Input: part model. Units: mm. Frame: model coordinates. Face numbers are marked on the shaded views. A direction names the side the tool comes from. Coordinates: 2 decimals unless noted, no trailing zeros. Write each loop counter-clockwise with the first axis right and the second up, starting at its lowest first coordinate (ties: lowest second). Pieces come first, ordered by that corner, then holes. Notation, with made-up numbers: (52.5, 79.25) - (63.5, 79.25) arc R14 cw to (63.5, 92.25) - close; hole circle Ø11 at (58.5, -35). An arc over 180 degrees is marked (long way). Put each result on its own line as item: value. Start each with the question number.
1. Pin query (flat end, axial travel): pin 1 (6 mm diameter, centred on x = -10, y = 9.5, fed in from -Z); pin 2 (3 mm diameter, centred on x = 17.5, z = 0, fed in from +Y); pin 3 (5 mm diameter, centred on x = 8, z = -10, fed in from +Y); pin 4 (5 mm diameter, centred on y = 6.5, z = 7.5, fed in from +X). Return the tip coordinate at first contact, or that it passes through.
2. Cut plane B-B, the plane x = -17. Return loops of the section in (y, z).
3. Access query for the marked faces 1 and 2. Directions: +Z, -Z, +X, -X, +Y, -Y. A direction counts if a zero-diameter tool reaches every point of the face in a straight line with its end or side. Return the directions, or none.
4. Cut plane A-A, the plane z = 0. Return loops of the section in (x, y), and give its area (3 significant figures).
5. Cut plane D-D, the plane z = 11.5. Return loops of the section in (x, y).
6. Cut plane C-C, the plane x = -4.5. Return loops of the section in (y, z), and give its area (3 significant figures).
7. Line query: line 1 (Y direction, x = -5, z = -10); line 2 (Z direction, x = 17.5, y = 0.75); line 3 (Y direction, x = 18.5, z = 5). Output: solid intervals per line, ascending.
from build123d import *

# Parameters (mm, degrees)
SKETCH_1_R      = 16.1
EXTRUDE_1_DEPTH = 1
SKETCH_2_R      = 13.5
EXTRUDE_2_DEPTH = 9
HOLE_WIZARD_1_D = 4
FILLET_1_R      = 10


with BuildPart() as part:
    # 草图1 → 凸台-拉伸1 (new body)
    with BuildSketch(Plane(origin=(0, 0, 0), x_dir=(1, 0, 0), z_dir=(0, 1, 0))):
        with BuildLine():
            Line((-23.5, 16.1), (-23.5, -16.1))
            Line((-23.5, -16.1), (0, -16.1))
            ThreePointArc((0, -16.1), (-16.1, 0), (0, 16.1))
            Line((0, 16.1), (-23.5, 16.1))
        make_face()
        Circle(SKETCH_1_R)
        with BuildLine():
            ThreePointArc((16.1, 0), (11.384419177, -11.384419177), (0, -16.1))
            Line((0, -16.1), (23.5, -16.1))
            Line((23.5, -16.1), (23.5, 16.1))
            Line((23.5, 16.1), (0, 16.1))
            ThreePointArc((0, 16.1), (11.384419177, 11.384419177), (16.1, 0))
        make_face()
    extrude(amount=EXTRUDE_1_DEPTH)

    # 草图2 → 凸台-拉伸2 (add)
    with BuildSketch(Plane(origin=(0, 1, 0), x_dir=(1, 0, 0), z_dir=(0, 1, 0))):
        with Locations(Location((0, 0, 0), (0, 0, 270))):
            Circle(SKETCH_2_R)
    extrude(amount=EXTRUDE_2_DEPTH)

    # 草图3 → 旋转1 (revolve)
    with BuildSketch(Plane.ZY):
        with BuildLine():
            Line((0, 15), (0, 10))
            Line((0, 10), (5, 10))
            ThreePointArc((5, 10), (3.535533906, 13.535533906), (0, 15))
        make_face()
    revolve(axis=Axis((0, 15, 0), (0, -1, 0)))

    # 孔1 (through all)
    with Locations(Plane(origin=(0, 1, 0), x_dir=(1, 0, 0), z_dir=(0, 1, 0))):
        with Locations((-17.5, 0), (17.5, 0)):
            Hole(HOLE_WIZARD_1_D / 2)

    # 圆角1
    fillet_1_edges = [part.edges().sort_by_distance(p)[0] for p in [
        (-23.5, 0.5, 16.1),
        (-23.5, 0.5, -16.1),
        (23.5, 0.5, -16.1),
        (23.5, 0.5, 16.1),
    ]]
    fillet(fillet_1_edges, radius=FILLET_1_R)


solid = part.part
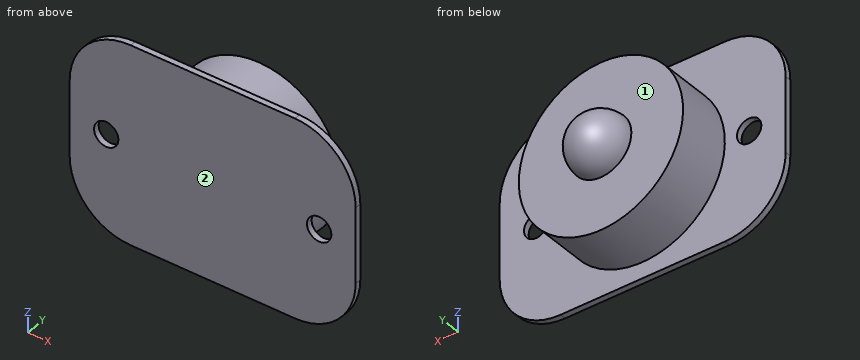
Report:
1. pin 1: stops at z = -11.54
1. pin 2: passes through
1. pin 3: stops at y = 10
1. pin 4: stops at x = 12.54
2. outline: (0, -15.47) - (1, -15.47) - (1, -1.94) - (0, -1.94) - close; (0, 1.94) - (1, 1.94) - (1, 15.47) - (0, 15.47) - close
3. face 1: +Y
3. face 2: +Z, -Z, +X, -X, -Y
4. outline: (-23.5, 0) - (-19.5, 0) - (-19.5, 1) - (-23.5, 1) - close; (-15.5, 0) - (15.5, 0) - (15.5, 1) - (13.5, 1) - (13.5, 10) - (5, 10) arc R5 ccw to (-5, 10) - (-13.5, 10) - (-13.5, 1) - (-15.5, 1) - close; (19.5, 0) - (23.5, 0) - (23.5, 1) - (19.5, 1) - close
4. area: 321 mm^2
5. outline: (-21.92, 0) - (21.92, 0) - (21.92, 1) - (7.07, 1) - (7.07, 10) - (-7.07, 10) - (-7.07, 1) - (-21.92, 1) - close
6. outline: (0, -16.1) - (1, -16.1) - (1, -12.73) - (10, -12.73) - (10, -2.18) arc R2.18 ccw to (10, 2.18) - (10, 12.73) - (1, 12.73) - (1, 16.1) - (0, 16.1) - close
6. area: 269 mm^2
7. line 1: y = 0 to 10
7. line 2: z = -15.27 to -2, 2 to 15.27
7. line 3: y = 0 to 1
